Read the model definition and answer for the solid it produces. Units are mm, in the model's axes. A direction names the side the tool comes from. Coordinates: 2 decimals unless noted, no trailing zeros. Order: outer loops, then holes, each group sorted by start corner. A loop starts at its lowest first (then second) coordinate and runs counter-clockwise, first axis right, second up. Notation, with made-up numbers: (-38, 48.5) - (-23, 48.5) arc R15 cw to (-23, 63.5) - close; hole circle Ø4 at (33, 54.5). An arc over 180 degrees is marked (long way). Answer as a JSON object with one key per item and string values. Group by question number.
from build123d import *

# Parameters (mm, degrees)
F0_R     = 27.686
F1_DEPTH = 1.5875
F2_R     = 28.575
F3_DEPTH = 1.5875
F4_R     = 1.5875
F5_DEPTH = 3.176
F6_SIZE  = 0.127


with BuildPart() as f1:
    # F0 (on Front) → F1 (new body)
    with BuildSketch(Plane.XZ):
        Circle(F0_R)
    extrude(amount=F1_DEPTH)

    # F2 (on face) → F3 (join)
    with BuildSketch(Plane.XZ.offset(1.5875)):
        Circle(F2_R)
    extrude(amount=F3_DEPTH)

    # F4 (on face) → F5 (cut, through all)
    with BuildSketch(Plane.XZ.offset(3.175)):
        Circle(F4_R)
    extrude(amount=-F5_DEPTH, mode=Mode.SUBTRACT)

    # F6
    f6_edges = [f1.edges().sort_by_distance(p)[0] for p in [
        (-28.575, -3.175, 0),
        (-27.686, 0, 0),
        (-28.575, -1.5875, 0),
    ]]
    chamfer(f6_edges, length=F6_SIZE)


solid = f1.part
1. A cutting plane is placed at C-C on y = -0.75. Write down the section's boundary in (x, z) (1 decimal), and give its area (3 significant figures).
2. Given pin 1 (1 mm diameter, centred on x = 4, z = 19.5, fed in from +Y); pin 2 (1 mm diameter, centred on y = -0.5, z = 19.5, fed in from +X), each flat-ended and moving along its own axis, determine where each tip first touches the part or whether it passes through.
3. For a pull along Z with two mould halves and no side action, classify faces 3 (the cylindrical face through (-28.547, -2.372, 1.256)), 4 (the flat face through (0, 0, -6)), 5 (the cylindrical face through (-0.34, -1.61, -1.55)) as pulls with the +Z half, pulls with the -Z half, needs draft (parallel to the pull), parting line crosses it, or undercut.
4. For faces 1 (the cylindrical face through (14.884, -0.847, 23.345)), 2 (the flat face through (6, -3.175, 0)), determine the directions among +Z, -Z, +X, -X, +Y, -Y from which every point of the face is accessible in a straight line to the end or side of a thin tool.
5. Straight lines are drawn through the part: L1, parallel to Z at x = 0, y = -0.7; L2, parallel to Z at x = 0, y = -1.75 (1 decimal); L3, parallel to Z at x = -7.5, y = -1.2. For each, find the intervals that lie inside material, in ascending order.
Derived:
{
 "1": {"outline": "circle Ø55.4 at (0, 0); hole circle Ø3.2 at (0, 0)", "area": "2,400 mm2"},
 "2": {"pin 1": "stops at y = 0", "pin 2": "stops at x = 20.14"},
 "3": {"face 3": "parting line crosses it", "face 4": "needs draft", "face 5": "undercut"},
 "4": {"face 1": "+Y", "face 2": "+Z, -Z, +X, -X, -Y"},
 "5": {"L1": "z = -27.69 to -1.59, 1.59 to 27.69", "L2": "z = -28.6 to -1.6, 1.6 to 28.6", "L3": "z = -26.65 to 26.65"}
}
